from build123d import *

# Parameters (mm, degrees)
SKETCH1_W           = 168
SKETCH1_H           = 113
BOSS_EXTRUDE1_DEPTH = 20
BOSS_EXTRUDE4_DEPTH = 5


with BuildPart() as part:
    # Sketch1 → Boss-Extrude1 (new body)
    with BuildSketch(Plane(origin=(0, 0, 0), x_dir=(1, 0, 0), z_dir=(0, 1, 0))):
        Polygon((178, 0), (0, 0), (0, -5), (0, -123), (178, -123), align=None)
        with Locations((89, -61.5)):
            Rectangle(SKETCH1_W, SKETCH1_H, mode=Mode.SUBTRACT)
    extrude(amount=BOSS_EXTRUDE1_DEPTH)

    # Sketch2 → Boss-Extrude4 (add)
    with BuildSketch(Plane(origin=(0, 20, 0), x_dir=(1, 0, 0), z_dir=(0, 1, 0))):
        Polygon((183, 5), (0, 5), (-5, 5), (-5, -128), (183, -128), align=None)
    extrude(amount=-BOSS_EXTRUDE4_DEPTH)


solid = part.part
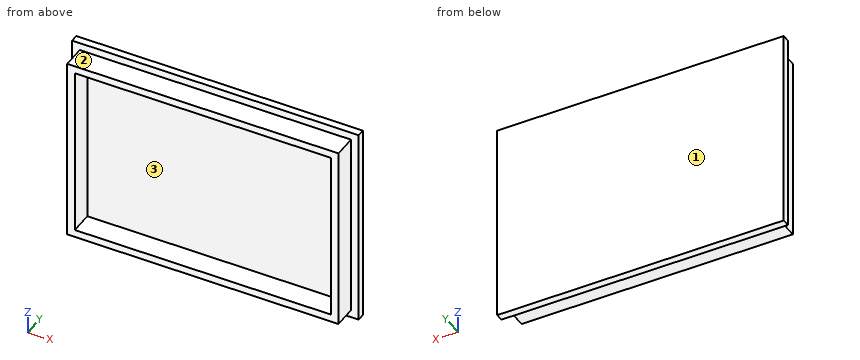
CAD build for the part. Positions are in the model's coordinates, mm. Face numbers are marked on the shaded views. Round coordinates to 2 decimals unless told otherwise and drop trailing zeros. Write each loop counter-clockwise with the first axis right and the second up, starting at its lowest first coordinate (ties: lowest second). Pieces come first, ordered by that corner, then holes. Notation, with made-up numbers: M 29,30 L 47,30 A12 cw 47,49 Z; hole C -32.75,74 d10. An arc over 180 degrees is marked long. Use a Markdown table: item, result. Add a question column.
1. Pull direction Z, two halves, no side cores. Call the marked faces 1, 2 and 3: released by +Z, released by -Z, zero draft, split by the parting line, or undercut.
2. Slice it at A-A on y = 12.5. Give the cut face in (x, z).
3. Drill centre lines: probe 1 along Z at (x, y) = (121, 5); probe 2 along X at (y, z) = (10.75, 48); probe 3 along Y at (x, z) = (139.5, 42). Where is each one in solid material? Low to high.
4. Slice it at C-C on z = 60.5. Give the cut face in (x, y).
5. Flat gauge pins, fed straight in: P1, Ø6, axis at y = 2, z = 30.5, coming from the +X side; P2, Ø1.5, axis at x = 89, y = 9.5, coming from the +Z side; P3, Ø8, axis at x = 82, y = 12, coming from the +Z side; P4, Ø12, axis at x = 105, y = 5.5, coming from the -Z side. Where does each tip first touch, or does it go through?
6. Slice it at B-B on x = 114.5. Give the cut face in (y, z), then the cut area to 3 significant figures.
Reply:
| question | item | result |
|---|---|---|
| 1 | face 1 | zero draft |
| 1 | face 2 | released by +Z |
| 1 | face 3 | undercut |
| 2 | outline | M 0,0 L 178,0 L 178,123 L 0,123 Z; hole M 5,5 L 173,5 L 173,118 L 5,118 Z |
| 3 | probe 1 | z = 0 to 5, 118 to 123 |
| 3 | probe 2 | x = 0 to 5, 173 to 178 |
| 3 | probe 3 | y = 15 to 20 |
| 4 | outline | M -5,15 L 0,15 L 0,0 L 5,0 L 5,15 L 173,15 L 173,0 L 178,0 L 178,15 L 183,15 L 183,20 L -5,20 Z |
| 5 | P1 | stops at x = 178 |
| 5 | P2 | stops at z = 123 |
| 5 | P3 | stops at z = 128 |
| 5 | P4 | stops at z = 0 |
| 6 | outline | M 0,0 L 15,0 L 15,-5 L 20,-5 L 20,128 L 15,128 L 15,123 L 0,123 L 0,118 L 15,118 L 15,5 L 0,5 Z |
| 6 | area | 815 mm^2 |
